from build123d import *

# Parameters (mm, degrees)
F0_R     = 1.5875
F1_DEPTH = 0.635


with BuildPart() as f1:
    # F0 (on Front) → F1 (new body, symmetric)
    with BuildSketch(Plane.XZ):
        with BuildLine():
            ThreePointArc((0.567515, 3.123868), (2.437467, 2.034547), (3.175, 0))
            ThreePointArc((3.175, 0), (2.344285, -2.14125), (0.286841, -3.162016))
            Line((0.286841, -3.162016), (21.143647, -1.27))
            ThreePointArc((21.143647, -1.27), (22.413647, 0), (21.143647, 1.27))
            Line((21.143647, 1.27), (0.567515, 3.123868))
        make_face()
        with BuildLine():
            ThreePointArc((0.286841, -3.162016), (2.344285, -2.14125), (3.175, 0))
            ThreePointArc((3.175, 0), (2.437467, 2.034547), (0.567515, 3.123868))
            Line((0.567515, 3.123868), (0, 3.175))
            ThreePointArc((0, 3.175), (-3.171752, -0.143567), (0.286841, -3.162016))
        make_face()
        Circle(F0_R, mode=Mode.SUBTRACT)
    extrude(amount=F1_DEPTH, both=True)


solid = f1.part
Geometry check sheet. Reference: the model listing, model coordinates, mm. Coordinates: 2 decimals unless noted, no trailing zeros. Order: outer loops, then holes, each group sorted by start corner. A loop starts at its lowest first (then second) coordinate and runs counter-clockwise, first axis right, second up. Notation, with made-up numbers: (63.5, 12.5) - (93.5, 12.5) arc R23 cw to (93.5, 35.5) - close; hole circle Ø6 at (-17, 88). An arc over 180 degrees is marked (long way). One line per item, written item: value.
(1) Thickness scan on probe 1 along X at (y, z) = (-0.5, 0.75); probe 2 along X at (y, z) = (0.6, 0.5); probe 3 along Z at (x, y) = (17.75, 0.3). Record the ranges inside material, lowest first. Write a range as from..to.
Data:
probe 1: x = -3.09..-1.4, 1.4..22.17
probe 2: x = -3.14..-1.51, 1.51..22.31
probe 3: z = -1.58..1.58
(2) Sectioned sample at C-C (x = 2). Enter the section's corners in (y, z) (3 decimals), and give its area (3 significant figures).
Data:
outline: (-0.635, -3.007) - (0.635, -3.007) - (0.635, 2.995) - (-0.635, 2.995) - close
area: 7.62 mm^2
(3) Release check for a two-part mould opening along Z. For faces 1 (the face through (22.413, -0.009, -0.028)), 2 (the face through (10.57, -0.01, -2.23)), 3 (the face through (9, 0.635, 0)), 4 (the face through (-0.34, 0.01, -1.55)) record: +Z half, -Z half, draft (parallel to the pull), parting line (faces both ways), or undercut.
Data:
face 1: parting line
face 2: -Z half
face 3: draft
face 4: undercut
(4) Sectioned sample at A-A (z = 0). Enter the section's corners in (x, y) (1 decimal).
Data:
outline: (-3.2, -0.6) - (-1.6, -0.6) - (-1.6, 0.6) - (-3.2, 0.6) - close; (1.6, -0.6) - (22.4, -0.6) - (22.4, 0.6) - (1.6, 0.6) - close
(5) Depth check by flat-ended pin: pin 1 Ø1.9 at (x, z) = (0, 0) entering from -Y. Enter the tip coordinate at first touch or a pass-through.
Data:
pin 1: passes through
(6) Sectioned sample at D-D (x = 20). Enter the section's corners in (y, z) (3 decimals).
Data:
outline: (-0.635, -1.374) - (0.635, -1.374) - (0.635, 1.373) - (-0.635, 1.373) - close
